Here's how the part is built. I have some questions about the finished solid (model axes, mm). A direction names the side the tool comes from. Coordinates: 2 decimals unless noted, no trailing zeros. Write each loop counter-clockwise with the first axis right and the second up, starting at its lowest first coordinate (ties: lowest second). Pieces come first, ordered by that corner, then holes.
Item 1: If we mould it in two halves opening along Z, with no side actions, what happens to faces 1 (the face through (7.676, 27.93, -30.363)), 2 (the face through (12.5, 32, -27)), 3 (the face through (0, 72, -38.1)), 4 (the face through (0, 69, -48.1))? For each: pulls with the +Z half, pulls with the -Z half, needs draft (parallel to the pull), parting line crosses it, or undercut.
Item 2: Please list where these lines run through material, in increasing order: line 1 (Y direction, x = 0, z = -8.5); line 2 (Z direction, x = 21, y = 65.5); line 3 (X direction, y = 36.5, z = -24.5).
Item 3: I'm going to push flat-ended pins straight in: P1, Ø8, axis at x = -17, z = -46, coming from the -Y side; P2, Ø5, axis at x = 11.5, y = 42.5, coming from the +Z side; P3, Ø1.7, axis at x = -9, z = -23.5, coming from the +Y side; P4, Ø10.5, axis at y = 6, z = -28.5, coming from the -X side. Where does each tip first touch, or does it pass through?
Item 4: For faces 5 (the face through (12.5, 10, -31)), 6 (the face through (-12.5, 10, -31)), 7 (the face through (-10, 20.65, -28)), 8 (the face through (10, 25.4, -27)), which set-ups out of +Z, -Z, +X, -X, +Y, -Y let a thin tool reach every point of the face, with its end or its side?
Item 5: I want a section at B-B (y = 57.5). Please give me the cut outline in (x, z) (1 decimal).
Item 6: I want a section at D-D (x = -14). Please give me the cut outline in (y, z), and give its area (3 significant figures).
Item 7: I want a section at C-C (z = -10). Please give me the cut outline in (x, y) (3 decimals), and give its area (3 significant figures).
from build123d import *

# Parameters (mm, degrees)
EXTRUDE1_DEPTH                   = 38.1
EXTRUDE2_DEPTH                   = 38.1
SKETCH4_W                        = 69.45
SKETCH4_H                        = 41.814012965
EXTRUDE3_DEPTH                   = 10
EXTRUDE4_DEPTH                   = 23.8125
CUT_EXTRUDE4_DEPTH               = 107.888880382
CUT_EXTRUDE4_DEPTH_BACK          = 107.888880382
F_25_0_1495_DIAMETER_HOLE1_D     = 3.7973
F_25_0_1495_DIAMETER_HOLE1_DEPTH = 26.9875
F_25_0_1495_DIAMETER_HOLE1_TIP   = 1.140824014
SKETCH11_R                       = 9.525
CUT_EXTRUDE2_DEPTH               = 30.1625
SKETCH12_R                       = 10.31875
CUT_EXTRUDE3_DEPTH               = 93.736926805
CUT_EXTRUDE5_START               = -12.5
CUT_EXTRUDE5_DEPTH               = 25


# Read off the part's stored shape, not the designer's step: Cut-Extrude5
with BuildPart() as part:
    # Sketch1 → Extrude1 (new body)
    with BuildSketch(Plane.XY):
        Polygon((12.5, 0), (-12.5, 0), (-12.5, 20.6502), (-6.9882, 20.6502), (-6.9882, 25.4), (-12.5, 25.4), (-12.5, 38.1), (-34.725, 38.1), (-34.725, 49.506590038), (34.725, 49.506590038), (34.725, 38.1), (12.5, 38.1), (12.5, 25.4), (6.9882, 25.4), (6.9882, 20.6502), (12.5, 20.6502), align=None)
    extrude(amount=-EXTRUDE1_DEPTH)

    # Sketch2 → Extrude2 (add)
    with BuildSketch(Plane.XY):
        with BuildLine():
            Line((-34.725, 60.107063342), (-34.725, 49.506590038))
            Line((-34.725, 49.506590038), (34.725, 49.506590038))
            Line((34.725, 49.506590038), (34.725, 60.107063342))
            Line((34.725, 60.107063342), (6.151391783, 70.643423952))
            ThreePointArc((6.151391783, 70.643423952), (0, 71.741434289), (-6.151391783, 70.643423952))
            Line((-6.151391783, 70.643423952), (-34.725, 60.107063342))
        make_face()
    extrude(amount=-EXTRUDE2_DEPTH)

    # Sketch4 → Extrude3 (add)
    with BuildSketch(Plane(origin=(0, 0, -38.1), x_dir=(-1, 0, 0), z_dir=(0, 0, -1))):
        with Locations((0, 59.007006483)):
            Rectangle(SKETCH4_W, SKETCH4_H)
    extrude(amount=EXTRUDE3_DEPTH)

    # Sketch13 → Extrude4 (add)
    with BuildSketch(Plane(origin=(0, 0, -38.1), x_dir=(-1, 0, 0), z_dir=(0, 0, -1))):
        Polygon((12.5, 38.1), (-12.5, 38.1), (-12.5, 25.4), (-6.9882, 25.4), (-6.9882, 20.6502), (-12.5, 20.6502), (-12.5, 0), (12.5, 0), (12.5, 20.6502), (6.9882, 20.6502), (6.9882, 25.4), (12.5, 25.4), align=None)
    extrude(amount=EXTRUDE4_DEPTH)

    # Sketch14 → Cut-Extrude4 (cut, two sides: drawn at the far end of the back side and taken through both)
    with BuildSketch(Plane(origin=(0, 0, 0), x_dir=(0, 0, -1), z_dir=(1, 0, 0)).offset(-CUT_EXTRUDE4_DEPTH_BACK)):
        with BuildLine():
            Line((61.9125, 38.1), (43.1, 38.1))
            ThreePointArc((43.1, 38.1), (44.02993597, 35.85493597), (46.275, 34.925))
            Line((46.275, 34.925), (61.9125, 34.925))
            Line((61.9125, 34.925), (61.9125, 38.1))
        make_face()
    extrude(amount=CUT_EXTRUDE4_DEPTH + CUT_EXTRUDE4_DEPTH_BACK, mode=Mode.SUBTRACT)

    # #25 (0.1495) Diameter Hole1
    with Locations(Plane.XZ):
        with Locations((-7.9375, -30.1625), (7.9375, -30.1625)):
            Hole(F_25_0_1495_DIAMETER_HOLE1_D / 2, depth=F_25_0_1495_DIAMETER_HOLE1_DEPTH)
            with Locations((0, 0, -(F_25_0_1495_DIAMETER_HOLE1_DEPTH + F_25_0_1495_DIAMETER_HOLE1_TIP / 2))):  # 118° drill point
                Cone(0, F_25_0_1495_DIAMETER_HOLE1_D / 2, F_25_0_1495_DIAMETER_HOLE1_TIP, mode=Mode.SUBTRACT)

    # Sketch11 → Cut-Extrude2 (cut)
    with BuildSketch(Plane.XY):
        with Locations((0, 53.961434289)):
            Circle(SKETCH11_R)
    extrude(amount=-CUT_EXTRUDE2_DEPTH, mode=Mode.SUBTRACT)

    # Sketch12 → Cut-Extrude3 (cut, through all)
    with BuildSketch(Plane.XY.offset(-30.1625)):
        with Locations((0, 53.961434289)):
            Circle(SKETCH12_R)
    extrude(amount=-CUT_EXTRUDE3_DEPTH, mode=Mode.SUBTRACT)

    # Cut-Extrude5 outline → Cut-Extrude5 (cut)
    with BuildSketch(Plane(origin=(0, 0, 0), x_dir=(0, 0, -1), z_dir=(1, 0, 0)).offset(CUT_EXTRUDE5_START)):
        Polygon((61.9125, 34.925), (52.3875, 34.925), (61.9125, 0), align=None)
    extrude(amount=CUT_EXTRUDE5_DEPTH, mode=Mode.SUBTRACT)


solid = part.part
Answer:
1. face 1: undercut
1. face 2: needs draft
1. face 3: pulls with the +Z half
1. face 4: pulls with the -Z half
2. line 1: y = 0 to 44.44, 63.49 to 71.74
2. line 2: z = -48.1 to -38.1
2. line 3: x = -12.5 to 12.5
3. P1: stops at y = 38.1
3. P2: stops at z = 0
3. P3: stops at y = 69.91
3. P4: stops at x = -12.5
4. face 5: +Z, -Z, +X, -Y
4. face 6: +Z, -Z, -X, -Y
4. face 7: +Z, -Z, -X
4. face 8: +Z, -Z, +X
5. outline: (-34.7, -48.1) - (-9.7, -48.1) - (-9.7, -30.2) - (-8.8, -30.2) - (-8.8, 0) - (-34.7, 0) - close; (8.8, -30.2) - (9.7, -30.2) - (9.7, -48.1) - (34.7, -48.1) - (34.7, 0) - (8.8, 0) - close
6. outline: (38.1, -48.1) - (79.91, -48.1) - (79.91, -38.1) - (67.75, -38.1) - (67.75, 0) - (38.1, 0) - close
6. area: 1,550 mm2
7. outline: (-34.725, 38.1) - (-12.5, 38.1) - (-12.5, 25.4) - (-6.988, 25.4) - (-6.988, 20.65) - (-12.5, 20.65) - (-12.5, 0) - (12.5, 0) - (12.5, 20.65) - (6.988, 20.65) - (6.988, 25.4) - (12.5, 25.4) - (12.5, 38.1) - (34.725, 38.1) - (34.725, 60.107) - (6.151, 70.643) arc R17.78 ccw to (-6.151, 70.643) - (-34.725, 60.107) - close; hole circle Ø19.05 at (0, 53.961)
7. area: 2,580 mm2
